```python
from build123d import *

# Parameters (mm, degrees)
SKETCH2_R               = 50
BOSS_EXTRUDE1_DEPTH     = 150
SKETCH3_R               = 48
CUT_EXTRUDE1_DEPTH      = 150
SKETCH4_W               = 10
SKETCH4_H               = 10
BOSS_EXTRUDE2_DEPTH     = 3
SKETCH5_W               = 10
SKETCH5_H               = 10
BOSS_EXTRUDE3_DEPTH     = 3
SKETCH7_W               = 10
SKETCH7_H               = 10
BOSS_EXTRUDE5_DEPTH     = 3
SKETCH8_W               = 10
SKETCH8_H               = 10
BOSS_EXTRUDE6_DEPTH     = 3
SKETCH9_R               = 3.5
CUT_EXTRUDE2_DEPTH      = 200
SKETCH10_R              = 3.5
CUT_EXTRUDE3_DEPTH      = 200
CUT_EXTRUDE4_DEPTH      = 150
CUT_EXTRUDE4_DEPTH_BACK = 150
SKETCH11_W              = 35
SKETCH11_H              = 15
SKETCH12_R              = 48.5
CUT_EXTRUDE5_DEPTH      = 150


with BuildPart() as part:
    # Sketch2 → Boss-Extrude1 (new body)
    with BuildSketch(Plane(origin=(0, 0, 0), x_dir=(1, 0, 0), z_dir=(0, 1, 0))):
        with Locations(Location((0, 0, 0), (0, 0, 270))):
            Circle(SKETCH2_R)
    extrude(amount=BOSS_EXTRUDE1_DEPTH)

    # Sketch3 → Cut-Extrude1 (cut)
    with BuildSketch(Plane(origin=(0, 150, 0), x_dir=(1, 0, 0), z_dir=(0, 1, 0))):
        with Locations(Location((0, 0, 0), (0, 0, 270))):
            Circle(SKETCH3_R)
    extrude(amount=-CUT_EXTRUDE1_DEPTH, mode=Mode.SUBTRACT)

    # Sketch4 → Boss-Extrude2 (add)
    with BuildSketch(Plane(origin=(0, 150, 0), x_dir=(1, 0, 0), z_dir=(0, 1, 0))):
        with Locations((54.749371855, 0)):
            Rectangle(SKETCH4_W, SKETCH4_H)
    extrude(amount=-BOSS_EXTRUDE2_DEPTH)

    # Sketch5 → Boss-Extrude3 (add)
    with BuildSketch(Plane(origin=(0, 150, 0), x_dir=(1, 0, 0), z_dir=(0, 1, 0))):
        with Locations((-54.749371855, 0)):
            Rectangle(SKETCH5_W, SKETCH5_H)
    extrude(amount=-BOSS_EXTRUDE3_DEPTH)

    # Sketch7 → Boss-Extrude5 (add)
    with BuildSketch(Plane(origin=(0, 0, 0), x_dir=(1, 0, 0), z_dir=(0, 1, 0))):
        with Locations((-54.749371855, 0)):
            Rectangle(SKETCH7_W, SKETCH7_H)
    extrude(amount=BOSS_EXTRUDE5_DEPTH)

    # Sketch8 → Boss-Extrude6 (add)
    with BuildSketch(Plane(origin=(0, 0, 0), x_dir=(-1, 0, 0), z_dir=(0, -1, 0))):
        with Locations((-54.749371855, 0)):
            Rectangle(SKETCH8_W, SKETCH8_H)
    extrude(amount=-BOSS_EXTRUDE6_DEPTH)

    # Sketch9 → Cut-Extrude2 (cut)
    with BuildSketch(Plane.XZ):
        with Locations(Location((54.545191051, 0, 0), (0, 0, 270))):
            Circle(SKETCH9_R)
    extrude(amount=-CUT_EXTRUDE2_DEPTH, mode=Mode.SUBTRACT)

    # Sketch10 → Cut-Extrude3 (cut)
    with BuildSketch(Plane(origin=(0, 0, 0), x_dir=(-1, 0, 0), z_dir=(0, -1, 0))):
        with Locations(Location((54.586012061, 0, 0), (0, 0, 90))):
            Circle(SKETCH10_R)
    extrude(amount=-CUT_EXTRUDE3_DEPTH, mode=Mode.SUBTRACT)

    # Sketch11 → Cut-Extrude4 (cut, two sides: drawn at the far end of the back side and taken through both)
    with BuildSketch(Plane.XY.offset(-CUT_EXTRUDE4_DEPTH_BACK)):
        with Locations((0, 138.072258372)):
            Rectangle(SKETCH11_W, SKETCH11_H)
    extrude(amount=CUT_EXTRUDE4_DEPTH + CUT_EXTRUDE4_DEPTH_BACK, mode=Mode.SUBTRACT)

    # Sketch12 → Cut-Extrude5 (cut)
    with BuildSketch(Plane(origin=(0, 150, 0), x_dir=(1, 0, 0), z_dir=(0, 1, 0))):
        with Locations(Location((0, 0, 0), (0, 0, 270))):
            Circle(SKETCH12_R)
    extrude(amount=-CUT_EXTRUDE5_DEPTH, mode=Mode.SUBTRACT)


solid = part.part
```
The listing builds one solid part. Answer for the finished solid, in the listing's coordinates (mm). A direction names the side the tool comes from. Coordinates: 2 decimals unless noted, no trailing zeros. Write each loop counter-clockwise with the first axis right and the second up, starting at its lowest first coordinate (ties: lowest second). Pieces come first, ordered by that corner, then holes. Notation, with made-up numbers: M -40,-2 L 11,-2 A32 cw 11,28 Z; hole C -16.75,-35.5 d2. An arc over 180 degrees is marked long. Use a Markdown table: item, result. Add a question column.
1. Which of the six approach directions +Z, -Z, +X, -X, +Y, -Y give full straight-line access (tool end or side, diameter ignored) to faces 1 (the cylindrical face through (-51.116, 1.479, 0.456)), 2 (the flat face through (0, 145.572, 49))?
2. Section D-D (z = 12) is taken. Give the vertices of the cut face in (x, y).
3. Straight lines are drawn through the part: line 1 along X through (y, z) = (48, 0); line 2 along X through (y, z) = (97.5, -33). For each, find the intervals that lie inside material, in ascending order. Write a range as [from, to].
4. Section A-A (x = 0) is taken. Give the vertices of the cut face in (y, z).
5. Given P1, Ø1, axis at y = 23, z = 18.5, coming from the +X side; P2, Ø0.9, axis at x = 56.5, y = 1.5, coming from the -Z side; P3, Ø1, axis at x = 46.5, y = 82, coming from the -Z side; P4, Ø4, axis at x = 54.55, z = 0, coming from the +Y side, each flat-ended and moving along its own axis, determine where each tip first touches the part or whether it passes through.
6. Section C-C (x = 20) is taken. Give the vertices of the cut face in (y, z), plus the area to 3 significant figures.
7. For a pull along X with two mould halves and no side action, classify faces 3 (the flat face through (-31.3, 150, -37.3)), 4 (the flat face through (0, 130.572, 49)), 5 (the cylindrical face through (-44.36, 73.95, 23.07)) as +X half, -X half, draft (parallel to the pull), parting line (faces both ways), or undercut.
8. Section B-B (z = 0) is taken. Count the separate pieces of the cut face and the enclosed holes in it, plus the area to 3 significant figures.
Data:
| question | item | result |
|---|---|---|
| 1 | face 1 | +Y, -Y |
| 1 | face 2 | +Z, -Z |
| 2 | outline | M -48.54,0 L -46.99,0 L -46.99,150 L -48.54,150 Z; M 46.99,0 L 48.54,0 L 48.54,150 L 46.99,150 Z |
| 3 | line 1 | x = [-50, -48.5], [48.5, 50] |
| 3 | line 2 | x = [-37.56, -35.54], [35.54, 37.56] |
| 4 | outline | M 0,-50 L 130.57,-50 L 130.57,-48.5 L 0,-48.5 Z; M 0,48.5 L 130.57,48.5 L 130.57,50 L 0,50 Z; M 145.57,-50 L 150,-50 L 150,-48.5 L 145.57,-48.5 Z; M 145.57,48.5 L 150,48.5 L 150,50 L 145.57,50 Z |
| 5 | P1 | stops at x = 46.65 |
| 5 | P2 | stops at z = -5 |
| 5 | P3 | stops at z = -19.6 |
| 5 | P4 | passes through |
| 6 | outline | M 0,-45.83 L 150,-45.83 L 150,-44.18 L 0,-44.18 Z; M 0,44.18 L 150,44.18 L 150,45.83 L 0,45.83 Z |
| 6 | area | 492 mm2 |
| 7 | face 3 | draft |
| 7 | face 4 | undercut |
| 7 | face 5 | parting line |
| 8 | separate pieces | 6 |
| 8 | enclosed holes | 0 |
| 8 | area | 483 mm2 |
